```python
from build123d import *

# Parameters (mm, degrees)
BOSS_EXTRUDE1_DEPTH            = 22.5
CUT_EXTRUDE1_DEPTH             = 36
CBORE_FOR_M3_SHCS1_D           = 3.4
CBORE_FOR_M3_SHCS1_DEPTH       = 5
CBORE_FOR_M3_SHCS1_CBORE_D     = 6.5
CBORE_FOR_M3_SHCS1_CBORE_DEPTH = 3
CBORE_FOR_M3_SHCS1_TIP         = 1.021463052
M3X0_5_TAPPED_HOLE1_D          = 2.5
M3X0_5_TAPPED_HOLE1_DEPTH      = 25.54449211
M3X0_5_TAPPED_HOLE1_TIP        = 0.751075774
FILLET2_R                      = 4
TOLERANCING_START              = -22.5
TOLERANCING_DEPTH              = 45


# Read off the part's stored shape, not the designer's step: Tolerancing
with BuildPart() as part:
    # Sketch1 → Boss-Extrude1 (new, symmetric)
    with BuildSketch(Plane(origin=(0, 0, 0), x_dir=(1, 0, 0), z_dir=(0, 1, 0))):
        with BuildLine():
            Line((-15, -26.997045256), (15, -26.997045256))
            ThreePointArc((15, -26.997045256), (35.338518717, 5), (15, 36.997045256))
            Line((15, 36.997045256), (-15, 36.997045256))
            ThreePointArc((-15, 36.997045256), (-35.338518717, 5), (-15, -26.997045256))
        make_face()
        with BuildLine():
            Line((-12.7, -21.997045256), (12.7, -21.997045256))
            ThreePointArc((12.7, -21.997045256), (0, 25.4), (-12.7, -21.997045256))
        make_face(mode=Mode.SUBTRACT)
    extrude(amount=BOSS_EXTRUDE1_DEPTH, both=True)

    # Sketch4 → Cut-Extrude1 (cut)
    with BuildSketch(Plane(origin=(0, 22.5, 0), x_dir=(1, 0, 0), z_dir=(0, 1, 0))):
        Polygon((-10, 36.997045256), (-10, 32.997045256), (-15, 32.997045256), (-15, 27.997045256), (15, 27.997045256), (15, 32.997045256), (10, 32.997045256), (10, 36.997045256), align=None)
    extrude(amount=-CUT_EXTRUDE1_DEPTH, mode=Mode.SUBTRACT)

    # CBORE for M3 SHCS1
    with Locations(Plane.XY.offset(26.997045256)):
        with Locations((0, 0), (0, 15), (0, -15)):
            CounterBoreHole(CBORE_FOR_M3_SHCS1_D / 2, CBORE_FOR_M3_SHCS1_CBORE_D / 2, CBORE_FOR_M3_SHCS1_CBORE_DEPTH, depth=CBORE_FOR_M3_SHCS1_DEPTH)
            with Locations((0, 0, -(CBORE_FOR_M3_SHCS1_DEPTH + CBORE_FOR_M3_SHCS1_TIP / 2))):  # 118° drill point
                Cone(0, CBORE_FOR_M3_SHCS1_D / 2, CBORE_FOR_M3_SHCS1_TIP, mode=Mode.SUBTRACT)

    # M3x0.5 Tapped Hole1
    with Locations(Plane(origin=(0, 0, -27.997045256), x_dir=(-1, 0, 0), z_dir=(0, 0, -1))):
        with Locations((0, 3.5), (0, -6.5)):
            Hole(M3X0_5_TAPPED_HOLE1_D / 2, depth=M3X0_5_TAPPED_HOLE1_DEPTH)
            with Locations((0, 0, -(M3X0_5_TAPPED_HOLE1_DEPTH + M3X0_5_TAPPED_HOLE1_TIP / 2))):  # 118° drill point
                Cone(0, M3X0_5_TAPPED_HOLE1_D / 2, M3X0_5_TAPPED_HOLE1_TIP, mode=Mode.SUBTRACT)

    # Fillet2
    fillet2_edges = [part.edges().sort_by_distance(p)[0] for p in [
        (10, -13.5, -34.997045256),
        (15, -13.5, -30.497045256),
        (-15, -13.5, -30.497045256),
        (-10, -13.5, -34.997045256),
    ]]
    fillet(fillet2_edges, radius=FILLET2_R)

    # Tolerancing outline → Tolerancing (cut)
    with BuildSketch(Plane(origin=(0, 0, 0), x_dir=(1, 0, 0), z_dir=(0, 1, 0)).offset(TOLERANCING_START)):
        with BuildLine():
            ThreePointArc((12.799707028, -21.997045256), (0, 25.45), (-12.799707028, -21.997045256))
            Line((-12.799707028, -21.997045256), (-12.7, -21.997045256))
            ThreePointArc((-12.7, -21.997045256), (0, 25.4), (12.7, -21.997045256))
            Line((12.7, -21.997045256), (12.799707028, -21.997045256))
        make_face()
    extrude(amount=TOLERANCING_DEPTH, mode=Mode.SUBTRACT)


solid = part.part
```
Verification items for the finished model (mm, model axes). A direction names the side the tool comes from. Give positions to 0.01 mm unless a question says otherwise; leave off trailing zeros. Loops run counter-clockwise (first coordinate to the right, second up) from the corner with the lowest first, then second, coordinate; pieces in that order, holes last. Notation, with made-up numbers: M 41,-23.75 L 66,-23.75 A26 cw 66,3.25 Z; hole C 69,-14.5 d4. An arc over 180 degrees is marked long. One line per question, with ' | ' between items.
Item 1: Section check B-B, the plane z = 16. Record the cut outline in (x, y), plus the area to 3 significant figures.
Completed:
outline: M -28.42,-22.5 L -19.79,-22.5 L -19.79,22.5 L -28.42,22.5 Z; M 19.79,-22.5 L 28.42,-22.5 L 28.42,22.5 L 19.79,22.5 Z | area: 777 mm^2
Item 2: Draft check along X on faces 6 (the face through (-8.859, -12.297, -34.969)), 7 (the face through (-4, 0, 26.997)), 8 (the face through (-13.859, -12.297, -30.462)). Enter one of: +X half, -X half, draft (parallel to the pull), parting line (faces both ways), or undercut.
Completed:
face 6: undercut | face 7: draft | face 8: undercut
Item 3: Section check D-D, the plane x = 0. State how many separate pieces and enclosed holes the cut face has, plus the area to 3 significant figures.
Completed:
separate pieces: 7 | enclosed holes: 0 | area: 329 mm^2
Item 4: Section check A-A, the plane x = -17. Record the cut outline in (y, z).
Completed:
outline: M -22.5,-35.98 L 22.5,-35.98 L 22.5,-18.94 L -22.5,-18.94 Z; M -22.5,18.94 L 22.5,18.94 L 22.5,25.98 L -22.5,25.98 Z
Item 5: Depth check by flat-ended pin: P1, Ø2, axis at x = 0.5, y = -16.5, coming from the +Z side; P2, Ø2.5, axis at x = 0, y = 15, coming from the -Z side; P3, Ø8, axis at x = -22, y = 0, coming from the -Z side. Enter the tip coordinate at first touch or a pass-through.
Completed:
P1: stops at z = 24 | P2: stops at z = -28 | P3: stops at z = -35.41
Item 6: Section check C-C, the plane y = -6.5. Record the cut outline in (x, z), plus the area to 3 significant figures.
Completed:
outline: M -15,-37 L -10,-37 L -10,-33 L -15,-33 L -15,-28 L -1.25,-28 L -1.25,-25.42 A25.45 cw -12.8,22 L 12.8,22 A25.45 cw 1.25,-25.42 L 1.25,-28 L 15,-28 L 15,-33 L 10,-33 L 10,-37 L 15,-37 A35.34 ccw 15,27 L -15,27 A35.34 ccw Z | area: 1,580 mm^2
Item 7: Thickness scan on line 1 (Y direction, x = 0, z = -26); line 2 (Y direction, x = 0, z = 22.7); line 3 (Y direction, x = 0, z = 26). Record the ranges inside material, lowest first. Write a range as [from, to].
Completed:
line 1: y = [-22.5, -7.75], [-5.25, 2.25], [4.75, 22.5] | line 2: y = [-22.5, -16.7], [-13.3, -1.7], [1.7, 13.3], [16.7, 22.5] | line 3: y = [-22.5, -18.25], [-11.75, -3.25], [3.25, 11.75], [18.25, 22.5]
Item 8: Tool access check on faces 1 (the face through (0.221, -13.314, 22.983)), 2 (the face through (-0.27, 2.28, -26.69)), 3 (the face through (3, 0, 21.997)), 4 (the face through (-10, 7, -35)), 5 (the face through (13.859, -12.297, -30.532)). Record the directions out of +Z, -Z, +X, -X, +Y, -Y that give a thin tool (end or side, any length) a straight path to the whole face; none if there is none.
Completed:
face 1: +Z | face 2: -Z | face 3: +Y, -Y | face 4: -Z, +Y | face 5: +Y
